Could you check a few things on this drawing? It's one solid part, dimensions in mm from its lowest x, y, z. A direction names the side the tool comes from. Coordinates: 2 decimals unless noted, no trailing zeros. Order: outer loops, then holes, each group sorted by start corner. A loop starts at its lowest first (then second) coordinate and runs counter-clockwise, first axis right, second up. Notation, with made-up numbers: (80.25, -11) - (111.25, -11) arc R11 cw to (111.25, 0) - close; hole circle Ø4 at (76, 51). An arc over 180 degrees is marked (long way). Return JSON: item names as keys, results as strings. Group by question number.
1) Imagine slicing it at A-A (y = 12.75). Write out the boundary of the cut face in (x, z), and give its area (3 significant figures).
2) Imagine slicing it at C-C (x = 36). Write out the boundary of the cut face in (y, z), and give its area (3 significant figures).
3) Which directions (+Z, -Z, +X, -X, +Y, -Y) give clear straight access to the entire face, cutting with the end or side of a thin tool? Please do the marked faces 1 and 2.
4) If we mould it in two halves opening along X, with no side actions, what happens to the marked faces 3, 4 and 5? For each: pulls with the +X half, pulls with the -X half, needs draft (parallel to the pull), parting line crosses it, or undercut.
5) If I drill on line 1 along X through (y, z) = (12.25, 12.5); line 2 along X through (y, z) = (4.25, 56.5), over which ranges is the centre line in solid material (lowest first)?
6) Imagine slicing it at B-B (z = 48). Write out the boundary of the cut face in (x, y).
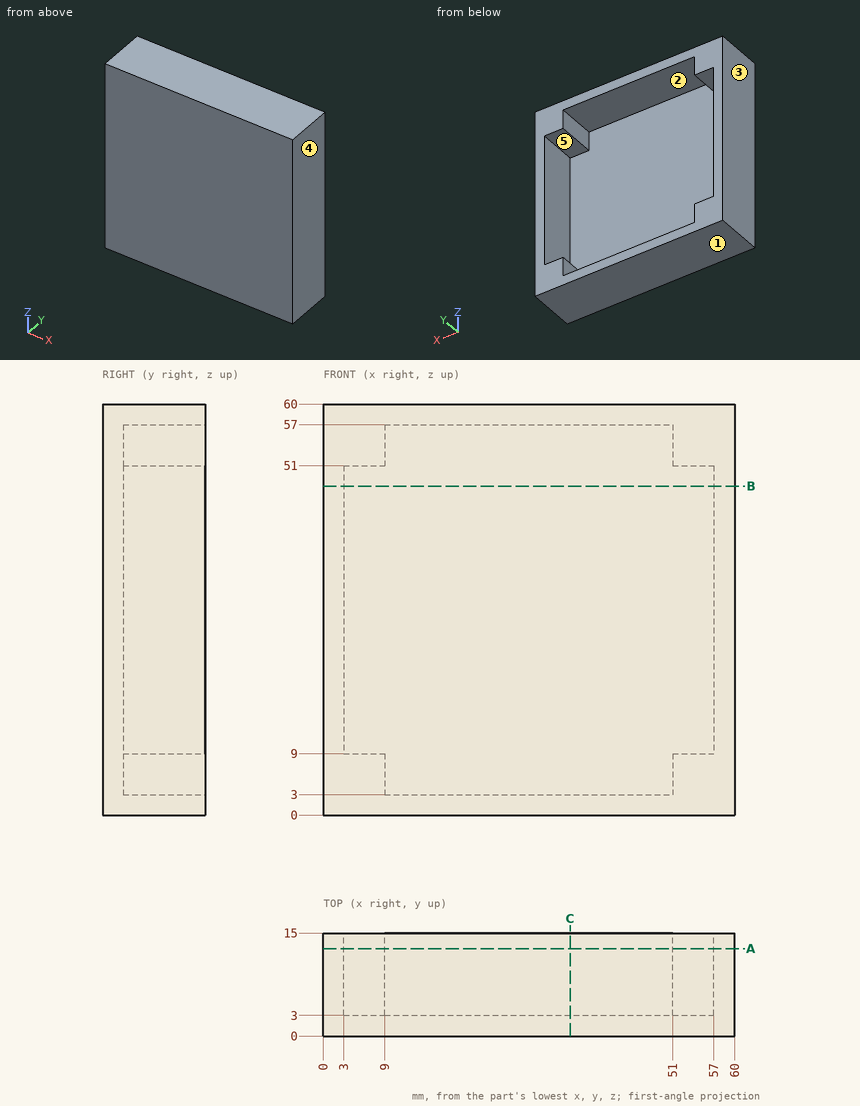
Calculated:
{
 "1": {"outline": "(0, 0) - (60, 0) - (60, 60) - (0, 60) - close; hole (3, 9) - (9, 9) - (9, 3) - (51, 3) - (51, 9) - (57, 9) - (57, 51) - (51, 51) - (51, 57) - (9, 57) - (9, 51) - (3, 51) - close", "area": "828 mm2"},
 "2": {"outline": "(0, 0) - (15, 0) - (15, 3) - (3, 3) - (3, 57) - (15, 57) - (15, 60) - (0, 60) - close", "area": "252 mm2"},
 "3": {"face 1": "-Z, +X, -X, +Y, -Y", "face 2": "+Y"},
 "4": {"face 3": "pulls with the -X half", "face 4": "pulls with the +X half", "face 5": "undercut"},
 "5": {"line 1": "0 to 3, 57 to 60", "line 2": "0 to 9, 51 to 60"},
 "6": {"outline": "(0, 0) - (60, 0) - (60, 15) - (57, 15) - (57, 3) - (3, 3) - (3, 15) - (0, 15) - close"}
}
